Design review of the part built by this model. Coordinates are the model's own, in mm. Face numbers are marked on the shaded views. A direction names the side the tool comes from. Coordinates: 2 decimals unless noted, no trailing zeros. Loops run counter-clockwise (first coordinate to the right, second up) from the corner with the lowest first, then second, coordinate; pieces in that order, holes last. Notation, with made-up numbers: M -32.75,65 L -25.75,65 A17 cw -25.75,88 Z; hole C 57,-31 d7. An arc over 180 degrees is marked long. Put each result on its own line as item: value. Start each with the question number.
(1) Take a section at A-A, the plane z = 0. Give the boundary of the cut face in (x, y) (3 decimals), then the cut area to 3 significant figures.
(2) Take a section at D-D, the plane z = 8.25. Give the boundary of the cut face in (x, y) (1 decimal).
(3) For the marked faces 1 and 2, list the 3-axis set-ups (+Z, -Z, +X, -X, +Y, -Y) from which the entire face can be reached by the end or side of a thin tool; tool diameter is ignored.
(4) For probe 1 along X at (y, z) = (-0.75, 7.5) (3 decimals); probe 2 along Y at (x, z) = (77.5, 1.25); probe 3 along Z at (x, y) = (14, 2), list the stretches that pass through material, from the lowest coordinate up. Write a range as [from, to].
(5) Clearance check with flat-ended pins moving along their axes: pin 1 (2 mm diameter, centred on y = 3.5, z = -7, fed in from -X) (3 decimals); pin 2 (1.5 mm diameter, centred on y = -2, z = -2, fed in from -X); pin 3 (10 mm diameter, centred on x = 33, z = 6.5, fed in from -Y); pin 4 (4 mm diameter, centred on x = 58, z = 0, fed in from -Y) (3 decimals). State where each tip first meets the part, or that it passes through.
(6) Take a section at C-C, the plane x = 37.5. Give the boundary of the cut face in (y, z) (3 decimals).
Autodesk Inventor part; units mm, degrees
ref_plane "dia1_XY" through (0, 3.175, 0) normal (1, 0, 0) x (0, 0, -1)
ref_plane "dia1_YZ" through (0, 3.175, 0) normal (0, 0, -1) x (0, 1, 0)
ref_plane "dia1_ZX" through (0, 3.175, 0) normal (0, 1, 0) x (1, 0, 0)
sketch "Sketch_1" plane through (0, 0, 0) normal (0, 0, 1) x (1, 0, 0)
  line L0 (110.4392, 0) -> (0, 0)
  line L1 (0, 0) -> (0, 3.175)
  line L2 (0, 3.175) -> (73.025, 3.175)
  line L3 (73.025, 3.175) -> (73.025, 9.6203)
  line L4 (73.025, 9.6203) -> (110.4392, 9.6203)
  line L5 (110.4392, 9.6203) -> (110.4392, 0)
  line L6 (110.4392, 0) -> (0, 0)
revolve "Revolution1" add sketch "Sketch_1" angle 360 about axis through (110.4392, 0, 0) along (1, 0, 0)
sketch "Sketch_3" plane through (0, 0, 0) normal (0, 0, 1) x (1, 0, 0)
  line L0 (0, 0) -> (-12.7, 0)
  line L1 (-12.7, 0) -> (-12.7, 2.634)
  line L2 (-12.7, 2.634) -> (-12.159, 3.175)
  line L3 (-12.159, 3.175) -> (0, 3.175)
  line L4 (0, 3.175) -> (0, 0)
  line L5 (0, 0) -> (-12.7, 0)
revolve "Revolution2" add sketch "Sketch_3" angle 360 about axis through (0, 0, 0) along (1, 0, 0)
thread "Thread1"
sketch "Sketch_30" plane through (0, 0, 0) normal (0, 0, 1) x (1, 0, 0)
  line L0 (0, 0) -> (-0.254, 0)
  line L1 (-0.254, 2.921) -> (0, 2.921)
  line L2 (0, 2.921) -> (0, 3.429)
  line L3 (0, 3.429) -> (-0.254, 3.429)
  line L4 (-0.254, 3.429) -> (-0.254, 2.921)
revolve "Revolution3" cut sketch "Sketch_30" angle 360 about axis through (0, 0, 0) along (1, 0, 0)
ref_plane "dia1_XY" through (0, 3.175, 0) normal (1, 0, 0) x (0, 0, -1)
ref_plane "dia1_YZ" through (0, 3.175, 0) normal (0, 0, -1) x (0, 1, 0)
ref_plane "dia1_ZX" through (0, 3.175, 0) normal (0, 1, 0) x (1, 0, 0)
ref_plane "dia12_XY" through (0, 0, 10.2235) normal (1, 0, 0) x (0, 0, -1)
ref_plane "dia12_YZ" through (0, 0, 10.2235) normal (0, 0, -1) x (0, 1, 0)
ref_plane "dia12_ZX" through (0, 0, 10.2235) normal (0, 1, 0) x (1, 0, 0)
ref_plane "dia1r_XY" through (0, 0, 10.9537) normal (1, 0, 0) x (0, 0, -1)
ref_plane "dia1r_YZ" through (0, 0, 10.9537) normal (0, 0, -1) x (0, 1, 0)
ref_plane "dia1r_ZX" through (0, 0, 10.9537) normal (0, 1, 0) x (1, 0, 0)
ref_plane "dia2_XY" through (0, -3.175, 0) normal (1, 0, 0) x (0, 0, -1)
ref_plane "dia2_YZ" through (0, -3.175, 0) normal (0, 0, -1) x (0, 1, 0)
ref_plane "dia2_ZX" through (0, -3.175, 0) normal (0, 1, 0) x (1, 0, 0)
ref_plane "dia22_XY" through (0, 0, -10.2235) normal (1, 0, 0) x (0, 0, -1)
ref_plane "dia22_YZ" through (0, 0, -10.2235) normal (0, 0, -1) x (0, 1, 0)
ref_plane "dia22_ZX" through (0, 0, -10.2235) normal (0, 1, 0) x (1, 0, 0)
ref_plane "dia2r_XY" through (0, 0, -10.9537) normal (1, 0, 0) x (0, 0, -1)
ref_plane "dia2r_YZ" through (0, 0, -10.9537) normal (0, 0, -1) x (0, 1, 0)
ref_plane "dia2r_ZX" through (0, 0, -10.9537) normal (0, 1, 0) x (1, 0, 0)
ref_plane "rl1_XY" through (-12.7, 0, 0) normal (1, 0, 0) x (0, 0, -1)
ref_plane "rl1_YZ" through (-12.7, 0, 0) normal (0, 0, -1) x (0, 1, 0)
ref_plane "rl1_ZX" through (-12.7, 0, 0) normal (0, 1, 0) x (1, 0, 0)
ref_plane "rl2_XY" through (0, 0, 0) normal (1, 0, 0) x (0, 0, -1)
ref_plane "rl2_YZ" through (0, 0, 0) normal (0, 0, -1) x (0, 1, 0)
ref_plane "rl2_ZX" through (0, 0, 0) normal (0, 1, 0) x (1, 0, 0)
ref_plane "rod_cp_XY" through (0, 0, 0) normal (1, 0, 0) x (0, 0, -1)
ref_plane "rod_cp_YZ" through (0, 0, 0) normal (0, 0, -1) x (0, 1, 0)
ref_plane "rod_cp_ZX" through (0, 0, 0) normal (0, 1, 0) x (1, 0, 0)
ref_plane "thd1_XY" through (-12.7, 3.175, 0) normal (1, 0, 0) x (0, 0, -1)
ref_plane "thd1_YZ" through (-12.7, 3.175, 0) normal (0, 0, -1) x (0, 1, 0)
ref_plane "thd1_ZX" through (-12.7, 3.175, 0) normal (0, 1, 0) x (1, 0, 0)
ref_plane "thd2_XY" through (-12.7, -3.175, 0) normal (1, 0, 0) x (0, 0, -1)
ref_plane "thd2_YZ" through (-12.7, -3.175, 0) normal (0, 0, -1) x (0, 1, 0)
ref_plane "thd2_ZX" through (-12.7, -3.175, 0) normal (0, 1, 0) x (1, 0, 0)
ref_plane "to_rod_clevis_XY" through (-16.764, 0, 0) normal (1, 0, 0) x (0, 0, -1)
ref_plane "to_rod_clevis_YZ" through (-16.764, 0, 0) normal (0, 0, -1) x (0, 1, 0)
ref_plane "to_rod_clevis_ZX" through (-16.764, 0, 0) normal (0, 1, 0) x (1, 0, 0)
properties part number "C-042-P0_rod" material "Stainless Steel"
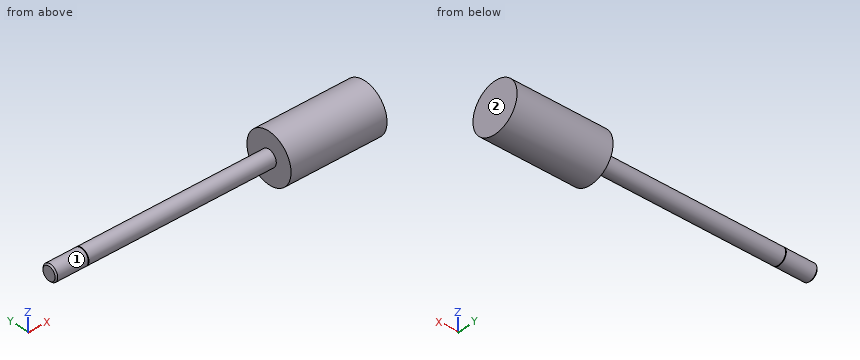
Computed values:
1. outline: M -12.7,-2.634 L -12.159,-3.175 L -0.254,-3.175 L -0.254,-2.921 L 0,-2.921 L 0,-3.175 L 73.025,-3.175 L 73.025,-9.62 L 110.439,-9.62 L 110.439,9.62 L 73.025,9.62 L 73.025,3.175 L 0,3.175 L 0,2.921 L -0.254,2.921 L -0.254,3.175 L -12.159,3.175 L -12.7,2.634 Z
1. area: 1,260 mm^2
2. outline: M 73,-4.9 L 110.4,-4.9 L 110.4,4.9 L 73,4.9 Z
3. face 1: -X
3. face 2: +Z, -Z, +X, +Y, -Y
4. probe 1: x = [73.025, 110.439]
4. probe 2: y = [-9.54, 9.54]
4. probe 3: z = [-2.47, 2.47]
5. pin 1: stops at x = 73.025
5. pin 2: stops at x = -12.7
5. pin 3: stops at y = -2.8
5. pin 4: stops at y = -3.175
6. outline: C 0,0 d6.35
